Source: CAD feature listing. Evaluate the final solid. Frame: model axes, mm. Face numbers are marked on the shaded views. Give positions to 0.01 mm unless a question says otherwise; leave off trailing zeros. Write each loop counter-clockwise with the first axis right and the second up, starting at its lowest first coordinate (ties: lowest second). Pieces come first, ordered by that corner, then holes.
```python
from build123d import *

# Parameters (mm, degrees)
BOSS_EXTRUDE1_DEPTH      = 3
BOSS_EXTRUDE1_DEPTH_BACK = 10
SKETCH1_R                = 10
SKETCH4_R                = 1.5
HOLE_DEPTH               = 20.973741561
HOLECIR_COUNT            = 5
SKETCH6_R                = 3
BEARINGHOLE_DEPTH        = 1.25
SKETCH7_R                = 1.5
SHAFTHOLE_DEPTH          = 17.248076982
SKETCH13_R               = 10
BOTTEN_HALF_DEPTH        = 10


with BuildPart() as part:
    # Sketch1 → Boss-Extrude1 (new, two sides: drawn at the far end of the back side and taken through both)
    with BuildSketch(Plane(origin=(0, 0, 0), x_dir=(1, 0, 0), z_dir=(0, 1, 0)).offset(-BOSS_EXTRUDE1_DEPTH_BACK)):
        with Locations(Location((0, 0, 0), (0, 0, 270))):
            Circle(SKETCH1_R)
    extrude(amount=BOSS_EXTRUDE1_DEPTH + BOSS_EXTRUDE1_DEPTH_BACK)

    # Sketch4 → hole (cut, through all)
    with BuildSketch(Plane(origin=(-3.352872105, -1.093066116, 1.887711608), x_dir=(-0.4486862613641547, -0.14627571033740308, -0.8816371449912632), z_dir=(0.8382180262940947, 0.2732665289126682, -0.47192790187872385))):
        with Locations(Location((0, 0, 0), (0, 0, 8.746528197))):
            Circle(SKETCH4_R)
    hole = extrude(amount=-HOLE_DEPTH, mode=Mode.SUBTRACT)

    # holecir: hole ×5 about axis
    holecir_axis = Axis((0, 0, 0), (0, 1, 0))
    for i in range(1, HOLECIR_COUNT):
        add(hole.rotate(holecir_axis, i * 360 / HOLECIR_COUNT), mode=Mode.SUBTRACT)

    # Sketch6 → bearinghole (cut, symmetric)
    with BuildSketch(Plane(origin=(0, -5, 0), x_dir=(-1, 0, 0), z_dir=(0, -1, 0))):
        with Locations(Location((0, 0, 0), (0, 0, 90))):
            Circle(SKETCH6_R)
    extrude(amount=BEARINGHOLE_DEPTH, both=True, mode=Mode.SUBTRACT)

    # Sketch7 → shafthole (cut, through all)
    with BuildSketch(Plane(origin=(0, -5, 0), x_dir=(-1, 0, 0), z_dir=(0, -1, 0))):
        with Locations(Location((0, 0, 0), (0, 0, 90))):
            Circle(SKETCH7_R)
    extrude(amount=SHAFTHOLE_DEPTH, mode=Mode.SUBTRACT)

    # Sketch13 → botten half (cut)
    with BuildSketch(Plane(origin=(0, -5, 0), x_dir=(-1, 0, 0), z_dir=(0, -1, 0))):
        with Locations(Location((0, 0, 0), (0, 0, 270))):
            Circle(SKETCH13_R)
    extrude(amount=-BOTTEN_HALF_DEPTH, mode=Mode.SUBTRACT)


solid = part.part
```
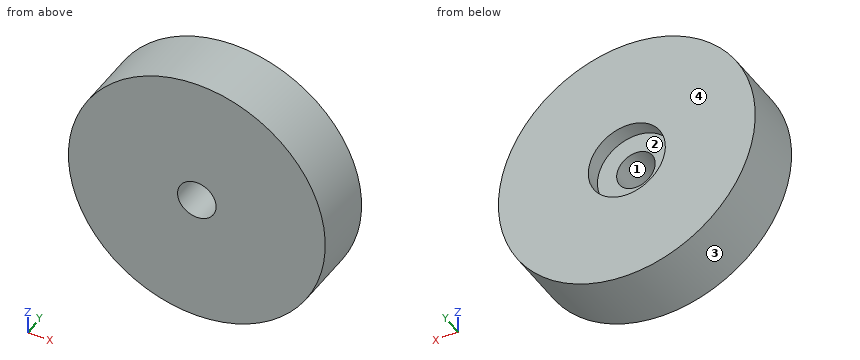
1. Pull-direction query (Z, two-part tool) for the marked faces 1, 2, 3 and 4; classes: pulls with the +Z half, pulls with the -Z half, needs draft (parallel to the pull), parting line crosses it, or undercut.
2. Line query: probe 1 along X at (y, z) = (-9.2, 0); probe 2 along X at (y, z) = (-5.65, 0). Output: solid intervals per line, ascending.
3. Section query A-A (z = 0). Return loops of the section in (x, y).
4. Section query B-B (x = 0). Return loops of the section in (y, z).
5. Section query D-D (x = 2.75). Return loops of the section in (y, z), plus the area to 3 significant figures.
6. Pin query (flat end, axial travel): P1, Ø3, axis at x = -4, y = -8.5, coming from the +Z side; P2, Ø2, axis at x = 1.5, y = -9, coming from the -Z side; P3, Ø1.5, axis at y = -8.5, z = -1, coming from the -X side. Return the tip coordinate at first contact, or that it passes through.
7. Section query C-C (y = -8.55). Return loops of the section in (x, z), plus the area to 3 significant figures.
The answers:
1. face 1: undercut
1. face 2: undercut
1. face 3: parting line crosses it
1. face 4: needs draft
2. probe 1: x = -10 to -1.5, 1.5 to 10
2. probe 2: x = -10 to -3, 3 to 10
3. outline: (-10, -10) - (-1.5, -10) - (-1.5, -6.25) - (-3, -6.25) - (-3, -5) - (-10, -5) - close; (1.5, -10) - (10, -10) - (10, -5) - (3, -5) - (3, -6.25) - (1.5, -6.25) - close
4. outline: (-10, -10) - (-5, -10) - (-5, -3) - (-6.25, -3) - (-6.25, -1.5) - (-10, -1.5) - close; (-10, 1.5) - (-6.25, 1.5) - (-6.25, 3) - (-5, 3) - (-5, 10) - (-10, 10) - close
5. outline: (-10, -9.61) - (-5, -9.61) - (-5, -1.2) - (-6.25, -1.2) - (-6.25, 1.2) - (-5, 1.2) - (-5, 9.61) - (-10, 9.61) - close
5. area: 93.1 mm2
6. P1: stops at z = 9.68
6. P2: stops at z = -9.99
6. P3: stops at x = -10
7. outline: circle Ø20 at (0, 0); hole circle Ø3 at (0, 0)
7. area: 307 mm2
